Verification items for the finished model (mm, model axes). A direction names the side the tool comes from. Give positions to 0.01 mm unless a question says otherwise; leave off trailing zeros. Order: outer loops, then holes, each group sorted by start corner. A loop starts at its lowest first (then second) coordinate and runs counter-clockwise, first axis right, second up. Notation, with made-up numbers: M 37.25,30 L 78.25,30 A26 ccw 78.25,46 Z; hole C -3.75,-19.75 d7. An arc over 180 degrees is marked long. Answer as a JSON object with one key per item and string values.
```python
from build123d import *

# Parameters (mm, degrees)
SKETCH1_W           = 63.5
SKETCH1_H           = 11.43
BOSS_EXTRUDE1_DEPTH = 82.55
SKETCH2_W           = 45.72
SKETCH2_H           = 77.47
CUT_EXTRUDE1_DEPTH  = 5.08
SKETCH3_W           = 13.335
SKETCH3_H           = 70.104
CUT_EXTRUDE2_DEPTH  = 105.77307574
SKETCH4_W           = 1.905
SKETCH4_H           = 70.104
CUT_EXTRUDE3_DEPTH  = 5.08
FILLET1_R           = 5.08
FILLET2_R           = 5.08
FILLET3_R           = 1.27
SKETCH5_R           = 2.2479
CUT_EXTRUDE4_DEPTH  = 105.77307574
SKETCH6_W           = 70.104
SKETCH6_H           = 6.35
BOSS_EXTRUDE2_DEPTH = 0.508


with BuildPart() as part:
    # Sketch1 → Boss-Extrude1 (new body)
    with BuildSketch(Plane.XY):
        with Locations((31.75, 5.715)):
            Rectangle(SKETCH1_W, SKETCH1_H)
    extrude(amount=BOSS_EXTRUDE1_DEPTH)

    # Sketch2 → Cut-Extrude1 (cut)
    with BuildSketch(Plane(origin=(0, 11.43, 0), x_dir=(1, 0, 0), z_dir=(0, 1, 0))):
        with Locations((38.1, -41.275)):
            Rectangle(SKETCH2_W, SKETCH2_H)
    extrude(amount=-CUT_EXTRUDE1_DEPTH, mode=Mode.SUBTRACT)

    # Sketch3 → Cut-Extrude2 (cut, through all)
    with BuildSketch(Plane(origin=(0, 11.43, 0), x_dir=(1, 0, 0), z_dir=(0, 1, 0))):
        with Locations((6.6675, -41.275)):
            Rectangle(SKETCH3_W, SKETCH3_H)
    extrude(amount=-CUT_EXTRUDE2_DEPTH, mode=Mode.SUBTRACT)

    # Sketch4 → Cut-Extrude3 (cut)
    with BuildSketch(Plane(origin=(0, 11.43, 0), x_dir=(1, 0, 0), z_dir=(0, 1, 0))):
        with Locations((14.2875, -41.275)):
            Rectangle(SKETCH4_W, SKETCH4_H)
    extrude(amount=-CUT_EXTRUDE3_DEPTH, mode=Mode.SUBTRACT)

    # Fillet1
    fillet1_edges = [part.edges().sort_by_distance(p)[0] for p in [
        (60.96, 8.89, 2.54),
        (60.96, 8.89, 80.01),
    ]]
    fillet(fillet1_edges, radius=FILLET1_R)

    # Fillet2
    fillet2_edges = [part.edges().sort_by_distance(p)[0] for p in [
        (63.5, 5.715, 82.55),
        (63.5, 5.715, 0),
    ]]
    fillet(fillet2_edges, radius=FILLET2_R)

    # Fillet3
    fillet3_edges = [part.edges().sort_by_distance(p)[0] for p in [
        (15.24, 8.89, 6.223),
        (15.24, 8.89, 76.327),
    ]]
    fillet(fillet3_edges, radius=FILLET3_R)

    # Sketch5 → Cut-Extrude4 (cut, through all)
    with BuildSketch(Plane.XY.offset(82.55)):
        with Locations((6.35, 5.715)):
            Circle(SKETCH5_R)
    extrude(amount=-CUT_EXTRUDE4_DEPTH, mode=Mode.SUBTRACT)

    # Sketch6 → Boss-Extrude2 (add)
    with BuildSketch(Plane.ZY.offset(-13.335)):
        with Locations((41.275, 3.175)):
            Rectangle(SKETCH6_W, SKETCH6_H)
    extrude(amount=BOSS_EXTRUDE2_DEPTH)


solid = part.part
```
Q1. Gauge pin test, flat ends, axial feed: pin 1 Ø4 at (y, z) = (9.5, 38.5) entering from -X; pin 2 Ø2 at (x, z) = (52, 59) entering from +Y; pin 3 Ø1.2 at (y, z) = (9.5, 79) entering from +X; pin 4 Ø4 at (x, y) = (6.35, 5.715) entering from -Z. Record the tip position at first contact, or that the pin passes through.
Resolved:
{"pin 1": "stops at x = 60.96", "pin 2": "stops at y = 6.35", "pin 3": "stops at x = 63.41", "pin 4": "passes through"}
Q2. Tool access check on faces 1 (the face through (59.511, 8.854, 78.482)), 2 (the face through (63.5, 6, 41)), 3 (the face through (12.827, 3, 41)), 4 (the face through (60.96, 9, 42)). Record the directions out of +Z, -Z, +X, -X, +Y, -Y that give a thin tool (end or side, any length) a straight path to the whole face; none if there is none.
Resolved:
{"face 1": "+Y", "face 2": "+Z, -Z, +X, +Y, -Y", "face 3": "-X, +Y, -Y", "face 4": "-X, +Y"}
Q3. Section check C-C on x = 50.5. Record the cut outline in (y, z).
Resolved:
{"outline": "M 0,0 L 11.43,0 L 11.43,2.54 L 6.35,2.54 L 6.35,80.01 L 11.43,80.01 L 11.43,82.55 L 0,82.55 Z"}
Q4. Release check for a two-part mould opening along Z. For faces 5 (the face through (15.24, 9, 4)), 6 (the face through (61.972, 5.795, 1.449)), 7 (the face through (39, 0, 41)) record: +Z half, -Z half, draft (parallel to the pull), parting line (faces both ways), or undercut.
Resolved:
{"face 5": "undercut", "face 6": "-Z half", "face 7": "draft"}
Q5. Section check D-D on z = 35. Record the cut outline in (x, y).
Resolved:
{"outline": "M 12.83,0 L 63.5,0 L 63.5,11.43 L 60.96,11.43 L 60.96,6.35 L 12.83,6.35 Z"}
Q6. Material ranges on L1, parallel to Z at x = 45.5, y = 8.5; L2, parallel to Z at x = 11, y = 4.75; L3, parallel to Y at x = 15, z = 43.5, recorded low to high.
Resolved:
{"L1": "z = 0 to 2.54, 80.01 to 82.55", "L2": "z = 0 to 6.22, 76.33 to 82.55", "L3": "y = 0 to 6.35"}
Q7. Section check A-A on x = 6.35. Record the cut outline in (y, z), then the cut area to 3 significant figures.
Resolved:
{"outline": "M 0,0 L 3.47,0 L 3.47,6.22 L 0,6.22 Z; M 0,76.33 L 3.47,76.33 L 3.47,82.55 L 0,82.55 Z; M 7.96,0 L 11.43,0 L 11.43,6.22 L 7.96,6.22 Z; M 7.96,76.33 L 11.43,76.33 L 11.43,82.55 L 7.96,82.55 Z", "area": "86.3 mm²"}
Q8. Section check B-B on y = 2.25. Record the cut outline in (x, z).
Resolved:
{"outline": "M 0,0 L 58.42,0 A5.08 ccw 63.5,5.08 L 63.5,77.47 A5.08 ccw 58.42,82.55 L 0,82.55 L 0,76.33 L 12.83,76.33 L 12.83,6.22 L 0,6.22 Z"}
